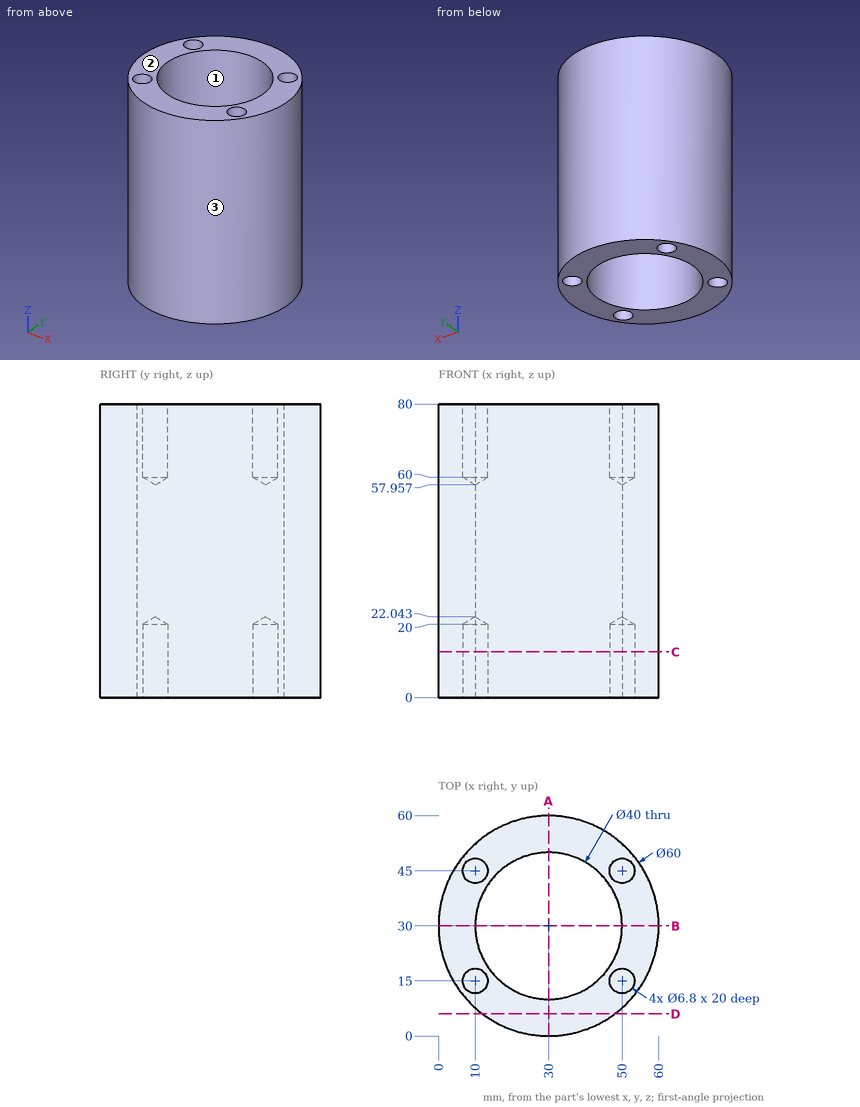
Print and shaded views of the part. All mm, measured from the part's lowest x, y and z. Coordinates: 2 decimals unless noted, no trailing zeros. Loops run counter-clockwise (first coordinate to the right, second up) from the corner with the lowest first, then second, coordinate; pieces in that order, holes last. Notation, with made-up numbers: (42.5, -15.75) - (55.5, -15.75) arc R33 cw to (55.5, 13.25) - close; hole circle Ø2 at (4.5, 43.25). An arc over 180 degrees is marked (long way). Use one line per item in the form item = value. Start each with the question number.
1) Band-saw the part on A-A (x = 30). Give the cut face in (y, z), and give its area (3 significant figures).
2) Drill centre lines: L1, parallel to X at y = 15, z = 7.5; L2, parallel to Y at x = 30, z = 24; L3, parallel to X at y = 23.5, z = 26. Where is each one in solid material? Low to high. Write a range as from..to.
3) Two-plate mould, pull along Y, no slides. Class the marked faces 1, 2 and 3: +Y half, -Y half, draft (parallel to the pull), parting line (faces both ways), or undercut.
4) Flat gauge pins, fed straight in: pin 1 (12 mm diameter, centred on x = 44, y = 24, fed in from +Z); pin 2 (3 mm diameter, centred on x = 51, z = 45, fed in from -Y); pin 3 (6 mm diameter, centred on x = 50, y = 15, fed in from -Z); pin 4 (5 mm diameter, centred on x = 14, z = 37, fed in from +Y). Where does each tip first touch, or does it go through?
5) Band-saw the part on C-C (z = 12.5). Give the cut face in (x, y).
6) Band-saw the part on D-D (y = 6). Give the cut face in (x, z), and give its area (3 significant figures).
Check values:
q1.outline = (0, 0) - (10, 0) - (10, 80) - (0, 80) - close; (50, 0) - (60, 0) - (60, 80) - (50, 80) - close
q1.area = 1,600 mm2
q2.L1 = 4.02..6.6, 13.4..16.77, 43.23..46.6, 53.4..55.98
q2.L2 = 0..10, 50..60
q2.L3 = 0.71..11.09, 48.91..59.29
q3.face_1 = undercut
q3.face_2 = draft
q3.face_3 = parting line
q4.pin_1 = 80
q4.pin_2 = 7.2
q4.pin_3 = 20.24
q4.pin_4 = 56.79
q5.outline = circle Ø60 at (30, 30); hole circle Ø6.8 at (10, 15); hole circle Ø6.8 at (10, 45); hole circle Ø40 at (30, 30); hole circle Ø6.8 at (50, 15); hole circle Ø6.8 at (50, 45)
q6.outline = (12, 0) - (48, 0) - (48, 80) - (12, 80) - close
q6.area = 2,880 mm2
